Part model, mm, in its own coordinate system. Face numbers are marked on the shaded views. Round coordinates to 2 decimals unless told otherwise and drop trailing zeros. Write each loop counter-clockwise with the first axis right and the second up, starting at its lowest first coordinate (ties: lowest second). Pieces come first, ordered by that corner, then holes.
1) Flat gauge pins, fed straight in: pin 1 (12 mm diameter, centred on x = 6.5, y = 0, fed in from -Z); pin 2 (3 mm diameter, centred on y = 5.5, z = 4.5, fed in from -X); pin 3 (2 mm diameter, centred on x = 17, z = 6.5, fed in from +Y). Where does each tip first touch, or does it go through?
2) Saw through at A-A on x = 0. Count the separate pieces of the cut face and the enclosed holes in it, and give its area (3 significant figures).
3) Saw through at D-D on z = 2. Write the cut outline in (x, y).
4) Pull direction X, two halves, no side cores. Call the marked faces 1, 2 and 3: +X half, -X half, draft (parallel to the pull), parting line (faces both ways), or undercut.
5) Saw through at C-C on z = 12. Write the cut outline in (x, y).
6) Drill centre lines: L1, parallel to Y at x = 1, z = 2.5; L2, parallel to Z at x = 7, y = -0.5; L3, parallel to X at y = -0.5, z = 11. Where is each one in solid material? Low to high.
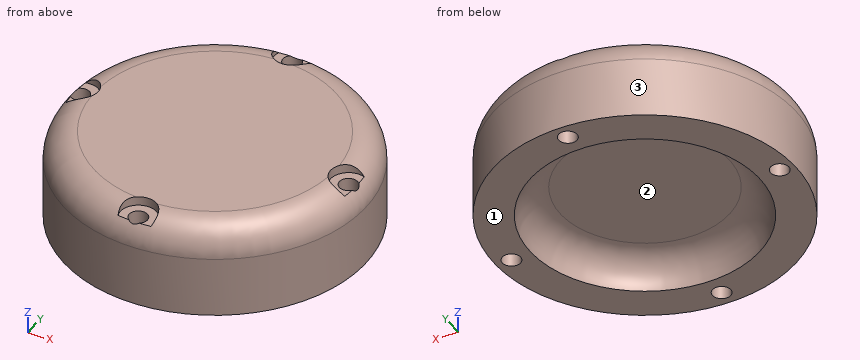
```python
from build123d import *

# Parameters (mm, degrees)
SKETCH1_R                                           = 25
SKETCH1_R_2                                         = 19
BOSS_EXTRUDE1_DEPTH                                 = 5
SKETCH2_R                                           = 25
BOSS_EXTRUDE2_DEPTH                                 = 10
FILLET1_R                                           = 5
CBORE_FOR_3_BINDING_HEAD_MACHINE_SCREW1_D           = 3.048
CBORE_FOR_3_BINDING_HEAD_MACHINE_SCREW1_CBORE_D     = 5.95376
CBORE_FOR_3_BINDING_HEAD_MACHINE_SCREW1_CBORE_DEPTH = 1.4986


with BuildPart() as part:
    # Sketch1 → Boss-Extrude1 (new body)
    with BuildSketch(Plane.XY):
        Circle(SKETCH1_R)
        Circle(SKETCH1_R_2, mode=Mode.SUBTRACT)
    extrude(amount=BOSS_EXTRUDE1_DEPTH)

    # Sketch2 → Boss-Extrude2 (add)
    with BuildSketch(Plane.XY.offset(5)):
        Circle(SKETCH2_R)
    extrude(amount=BOSS_EXTRUDE2_DEPTH)

    # Fillet1
    fillet1_edges = [part.edges().sort_by_distance(p)[0] for p in [
        (-25, 0, 15),
        (-19, 0, 5),
    ]]
    fillet(fillet1_edges, radius=FILLET1_R - 0.0001)  # a hair under: the kernel refuses the full size

    # CBORE for #3 Binding Head Machine Screw1 (through all)
    with Locations(Plane.XY.offset(15)):
        with Locations((0, 22.435050854), (0, -22.295918756), (22.400267829, 0), (-22.608965977, 0)):
            CounterBoreHole(CBORE_FOR_3_BINDING_HEAD_MACHINE_SCREW1_D / 2, CBORE_FOR_3_BINDING_HEAD_MACHINE_SCREW1_CBORE_D / 2, CBORE_FOR_3_BINDING_HEAD_MACHINE_SCREW1_CBORE_DEPTH)


solid = part.part
```
Completed:
1. pin 1: stops at z = 5
1. pin 2: stops at x = -24.68
1. pin 3: stops at y = 19.21
2. separate pieces: 3
2. enclosed holes: 0
2. area: 469 mm2
3. outline: circle Ø50 at (0, 0); hole circle Ø3.05 at (-22.61, 0); hole circle Ø37.17 at (0, 0); hole circle Ø3.05 at (0, -22.3); hole circle Ø3.05 at (0, 22.44); hole circle Ø3.05 at (22.4, 0)
4. face 1: draft
4. face 2: undercut
4. face 3: parting line
5. outline: circle Ø49.17 at (0, 0); hole circle Ø3.05 at (-22.61, 0); hole circle Ø3.05 at (0, -22.3); hole circle Ø3.05 at (0, 22.44); hole circle Ø3.05 at (22.4, 0)
6. L1: y = -24.98 to -23.45, -21.15 to -18.3, 18.3 to 21.29, 23.59 to 24.98
6. L2: z = 5 to 15
6. L3: x = -24.89 to -24.05, -21.17 to 20.96, 23.84 to 24.89
